Source: CAD feature listing. Evaluate the final solid. Frame: model axes, mm. A direction names the side the tool comes from. Give positions to 0.01 mm unless a question says otherwise; leave off trailing zeros. Loops run counter-clockwise (first coordinate to the right, second up) from the corner with the lowest first, then second, coordinate; pieces in that order, holes last.
```python
from build123d import *

# Parameters (mm, degrees)
F0_W     = 188
F0_H     = 185
F1_DEPTH = 20
F2_W     = 60
F2_H     = 89.5
F3_DEPTH = 25
F6_W     = 10
F6_H     = 20
F5_W     = 10
F5_H     = 2
F4_W     = 10
F4_H     = 20


with BuildPart() as f1:
    # F0 (on Top) → F1 (new body)
    with BuildSketch(Plane.XY):
        Rectangle(F0_W, F0_H)
    extrude(amount=F1_DEPTH)

    # F2 (on face) → F3 (cut)
    with BuildSketch(Plane.XY.offset(20)):
        with Locations((62, 45.75)):
            Rectangle(F2_W, F2_H)
        with Locations((0, 45.75)):
            Rectangle(F2_W, F2_H)
        with Locations((-62, 45.75)):
            Rectangle(F2_W, F2_H)
        with Locations((62, -45.75)):
            Rectangle(F2_W, F2_H)
        with Locations((0, -45.75)):
            Rectangle(F2_W, F2_H)
        with Locations((-62, -45.75)):
            Rectangle(F2_W, F2_H)
    extrude(amount=-F3_DEPTH, mode=Mode.SUBTRACT)

    # F6 (on face) → F8 section 0
    with BuildSketch(Plane.XZ.offset(-90.5)):
        with Locations((-62, 10)):
            Rectangle(F6_W, F6_H)
    # F5 (on Front) → F8 section 1
    with BuildSketch(Plane.XZ):
        with Locations((-62, 1)):
            Rectangle(F5_W, F5_H)
    loft()

    # F6 (on face) → F9 section 0
    with BuildSketch(Plane.XZ.offset(-90.5)):
        with Locations((0, 10)):
            Rectangle(F6_W, F6_H)
    # F5 (on Front) → F9 section 1
    with BuildSketch(Plane.XZ):
        with Locations((0, 1)):
            Rectangle(F5_W, F5_H)
    loft()

    # F6 (on face) → F10 section 0
    with BuildSketch(Plane.XZ.offset(-90.5)):
        with Locations((62, 10)):
            Rectangle(F6_W, F6_H)
    # F5 (on Front) → F10 section 1
    with BuildSketch(Plane.XZ):
        with Locations((62, 1)):
            Rectangle(F5_W, F5_H)
    loft()

    # F5 (on Front) → F11 section 0
    with BuildSketch(Plane.XZ):
        with Locations((62, 1)):
            Rectangle(F5_W, F5_H)
    # F4 (on face) → F11 section 1
    with BuildSketch(Plane(origin=(0, -90.5, 0), x_dir=(-1, 0, 0), z_dir=(0, 1, 0))):
        with Locations((-62, 10)):
            Rectangle(F4_W, F4_H)
    loft()

    # F4 (on face) → F12 section 0
    with BuildSketch(Plane(origin=(0, -90.5, 0), x_dir=(-1, 0, 0), z_dir=(0, 1, 0))):
        with Locations((0, 10)):
            Rectangle(F4_W, F4_H)
    # F5 (on Front) → F12 section 1
    with BuildSketch(Plane.XZ):
        with Locations((0, 1)):
            Rectangle(F5_W, F5_H)
    loft()

    # F4 (on face) → F13 section 0
    with BuildSketch(Plane(origin=(0, -90.5, 0), x_dir=(-1, 0, 0), z_dir=(0, 1, 0))):
        with Locations((62, 10)):
            Rectangle(F4_W, F4_H)
    # F5 (on Front) → F13 section 1
    with BuildSketch(Plane.XZ):
        with Locations((-62, 1)):
            Rectangle(F5_W, F5_H)
    loft()


solid = f1.part
```
(1) Section A-A, the plane x = -25. Return the cut outline in (y, z), then the cut area to 3 significant figures.
A:
outline: (-92.5, 0) - (-90.5, 0) - (-90.5, 20) - (-92.5, 20) - close; (-1, 0) - (1, 0) - (1, 20) - (-1, 20) - close; (90.5, 0) - (92.5, 0) - (92.5, 20) - (90.5, 20) - close
area: 120 mm2
(2) Reachability of faces 1 (the flat face through (-62.07, -45.123, 10.975)), 2 (the flat face through (-32, -46, 10)) from +Z, -Z, +X, -X, +Y, -Y: full face, straight path, thin tool, end or side. Return the list, or none.
A:
face 1: +Z
face 2: +Z, -Z
(3) Section B-B, the plane x = 2.5. Return the cut outline in (y, z), then the cut area to 3 significant figures.
A:
outline: (-92.5, 0) - (92.5, 0) - (92.5, 20) - (90.5, 20) - (1, 2.2) - (1, 20) - (-1, 20) - (-1, 2.2) - (-90.5, 20) - (-92.5, 20) - close
area: 2,110 mm2
(4) First-contact query: pin 1 (12 mm diameter, centred on x = 15, y = -67.5, fed in from -Z); pin 2 (5 mm diameter, centred on x = -0.5, y = -62.5, fed in from +Z). Flat tips, straight axial feed; report the tip coordinate or a pass-through.
A:
pin 1: passes through
pin 2: stops at z = 14.93
(5) Section C-C, the plane y = 9. Count the separate pieces of the cut face and the enclosed holes in it, then the cut area to 3 significant figures.
A:
separate pieces: 7
enclosed holes: 0
area: 274 mm2
(6) Ray query, line 1 along X through (y, z) = (62, 15); line 2 along Y through (x, z) = (68, 7.5); line 3 along Z through (x, y) = (60, 72.5). Return the intervals inside material, ascending.
A:
line 1: x = -94 to -92, -32 to -30, 30 to 32, 92 to 94
line 2: y = -92.5 to -90.5, -1 to 1, 90.5 to 92.5
line 3: z = 0 to 16.42
